```python
from build123d import *

# Parameters (mm, degrees)
F0_R     = 4.1
F0_W     = 42
F0_H     = 42
F0_W_2   = 30
F0_H_2   = 10
F1_DEPTH = 25
F0_R_2   = 9.7
F2_DEPTH = 6
F3_SIZE  = 5
F4_R     = 5
F5_R     = 12.5
F7_R     = 2.1
F6_R     = 2.1
F8_DEPTH = 25


with BuildPart() as f1:
    # F0 (on Top) → F1 (new body)
    with BuildSketch(Plane.XY):
        Polygon((-50, -30), (-50, -40), (50, -40), (50, -30), (50, 40), (-50, 40), align=None)
        with Locations((-35.5, -30.5)):
            Circle(F0_R, mode=Mode.SUBTRACT)
        with Locations((35.5, -30.5)):
            Circle(F0_R, mode=Mode.SUBTRACT)
        with Locations((-35.5, 30.5)):
            Circle(F0_R, mode=Mode.SUBTRACT)
        Rectangle(F0_W, F0_H, mode=Mode.SUBTRACT)
        with Locations((35.5, 30.5)):
            Circle(F0_R, mode=Mode.SUBTRACT)
        with Locations((-65, -35)):
            Rectangle(F0_W_2, F0_H_2)
        with Locations((65, -35)):
            Rectangle(F0_W_2, F0_H_2)
    extrude(amount=F1_DEPTH)

    # F0 (on Top) → F2 (join)
    with BuildSketch(Plane.XY):
        Rectangle(F0_W, F0_H)
        Circle(F0_R_2, mode=Mode.SUBTRACT)
    extrude(amount=F2_DEPTH)

    # F3
    f3_edges = [f1.edges().sort_by_distance(p)[0] for p in [
        (0, 21, 25),
        (-21, 0, 25),
        (0, -21, 25),
        (21, 0, 25),
    ]]
    chamfer(f3_edges, length=F3_SIZE)

    # F4
    f4_edges = [f1.edges().sort_by_distance(p)[0] for p in [
        (-50, -30, 12.5),
        (-50, 40, 12.5),
        (50, 40, 12.5),
        (50, -30, 12.5),
    ]]
    fillet(f4_edges, radius=F4_R)

    # F5
    f5_edges = [f1.edges().sort_by_distance(p)[0] for p in [
        (80, -35, 0),
        (-80, -35, 0),
    ]]
    fillet(f5_edges, radius=F5_R)

    # F7 (on face) + F6 (on face) → F8 (cut)
    with BuildSketch(Plane(origin=(0, -30, 0), x_dir=(-1, 0, 0), z_dir=(0, 1, 0))):
        with Locations((-67.5, 12.5)):
            Circle(F7_R)
    with BuildSketch(Plane(origin=(0, -30, 0), x_dir=(-1, 0, 0), z_dir=(0, 1, 0))):
        with Locations((67.5, 12.5)):
            Circle(F6_R)
    extrude(amount=-F8_DEPTH, mode=Mode.SUBTRACT)


solid = f1.part
```
Source: CAD feature listing. Evaluate the final solid. Frame: model axes, mm. A direction names the side the tool comes from. Coordinates: 2 decimals unless noted, no trailing zeros. Write each loop counter-clockwise with the first axis right and the second up, starting at its lowest first coordinate (ties: lowest second). Pieces come first, ordered by that corner, then holes. Notation, with made-up numbers: M 21.25,-21.5 L 36.25,-21.5 A27 ccw 36.25,9.5 Z; hole C -15,56.5 d9. An arc over 180 degrees is marked long. Answer as a JSON object with one key per item and string values.
1. Contact query for flat-ended pins moving along their axis: P1, Ø1, axis at x = -36, y = 0, coming from the -Z side; P2, Ø25, axis at x = 0, y = 0, coming from the +Z side; P3, Ø3, axis at y = 5, z = 14.5, coming from the +X side; P4, Ø12.5, axis at y = 9, z = 11.5, coming from the -X side. Output: stop coordinate, or through.
Evaluation:
{"P1": "z = 0", "P2": "z = 6", "P3": "x = 50", "P4": "x = -50"}
2. Access query for faces 4 (the flat face through (67, -30, 15)), 5 (the cylindrical face through (-69.44, -34.93, 11.7)), 6 (the flat face through (0, 21, 13)). Directions: +Z, -Z, +X, -X, +Y, -Y. A direction counts if a zero-diameter tool reaches every point of the face in a straight line with its end or side. Return the directions, or none.
Evaluation:
{"face 4": "+Z, -Z, +X, +Y", "face 5": "+Y, -Y", "face 6": "+Z"}
3. Cut plane D-D on x = 0. Output: boundary loops of the cut face in (y, z), plus the area to 3 significant figures.
Evaluation:
{"outline": "M -40,0 L -9.7,0 L -9.7,6 L -21,6 L -21,20 L -26,25 L -40,25 Z; M 9.7,0 L 40,0 L 40,25 L 26,25 L 21,20 L 21,6 L 9.7,6 Z", "area": "1,060 mm^2"}
4. Cut plane A-A on x = -35.5. Output: boundary loops of the cut face in (y, z), plus the area to 3 significant figures.
Evaluation:
{"outline": "M -40,0 L -34.6,0 L -34.6,25 L -40,25 Z; M -26.4,0 L 26.4,0 L 26.4,25 L -26.4,25 Z; M 34.6,0 L 40,0 L 40,25 L 34.6,25 Z", "area": "1,590 mm^2"}
5. Cut plane C-C on z = 2.5. Output: boundary loops of the cut face in (x, y), plus the area to 3 significant figures.
Evaluation:
{"outline": "M -75,-40 L 75,-40 L 75,-30 L 55,-30 A5 cw 50,-25 L 50,35 A5 ccw 45,40 L -45,40 A5 ccw -50,35 L -50,-25 A5 cw -55,-30 L -75,-30 Z; hole C -35.5,-30.5 d8.2; hole C -35.5,30.5 d8.2; hole C 0,0 d19.4; hole C 35.5,-30.5 d8.2; hole C 35.5,30.5 d8.2", "area": "7,990 mm^2"}
6. Cut plane B-B on y = 0. Output: boundary loops of the cut face in (x, z), plus the area to 3 significant figures.
Evaluation:
{"outline": "M -50,0 L -9.7,0 L -9.7,6 L -21,6 L -21,20 L -26,25 L -50,25 Z; M 9.7,0 L 50,0 L 50,25 L 26,25 L 21,20 L 21,6 L 9.7,6 Z", "area": "1,560 mm^2"}
7. Ray query, L1, parallel to Y at x = 35.5, z = 17.25; L2, parallel to X at y = -2, z = 12.25; L3, parallel to Y at x = -38, z = 22.5. Return the intervals inside material, ascending.
Evaluation:
{"L1": "-40 to -34.6, -26.4 to 26.4, 34.6 to 40", "L2": "-50 to -21, 21 to 50", "L3": "-40 to -33.75, -27.25 to 27.25, 33.75 to 40"}
8. Draft query along Y for faces 1 (the flat face through (24, 0, 23)), 2 (the flat face through (-50, 5, 12)), 3 (the cylindrical face through (-51, -28, 13)). Return one class per face: released by +Y, released by -Y, zero draft, split by the parting line, or undercut.
Evaluation:
{"face 1": "undercut", "face 2": "zero draft", "face 3": "released by +Y"}
